The model under review builds one solid part; all positions refer to its coordinate system, in mm. A direction names the side the tool comes from. Round coordinates to 2 decimals unless told otherwise and drop trailing zeros. Use one line per item in the form item = value.
from build123d import *

# Parameters (mm, degrees)
SKETCH1_R            = 180
SKETCH1_R_2          = 110
BOTTOM_ANNULUS_DEPTH = 10
SKETCH3_R            = 180
SKETCH3_R_2          = 110
ANNULUS_PLENUM_DEPTH = 12
SKETCH4_R            = 180
SKETCH4_R_2          = 110
TOP_ANNULUS_DEPTH    = 10
SKETCH8_R            = 6.6
CUT_EXTRUDE1_DEPTH   = 75
SKETCH6_R            = 18
SKETCH6_R_2          = 10
BOSS_EXTRUDE6_DEPTH  = 6.871206759
SKETCH10_R           = 10
SKETCH10_R_2         = 7
BOSS_EXTRUDE7_DEPTH  = 33.989306272


with BuildPart() as part:
    # Sketch1 → Bottom Annulus (new body)
    with BuildSketch(Plane.XY):
        Circle(SKETCH1_R)
        Circle(SKETCH1_R_2, mode=Mode.SUBTRACT)
    extrude(amount=BOTTOM_ANNULUS_DEPTH)

    # Sketch3 → Annulus Plenum (add)
    with BuildSketch(Plane.XY.offset(10)):
        Circle(SKETCH3_R)
        Circle(SKETCH3_R_2, mode=Mode.SUBTRACT)
    extrude(amount=ANNULUS_PLENUM_DEPTH)

    # Sketch4 → Top annulus (add)
    with BuildSketch(Plane.XY.offset(22)):
        Circle(SKETCH4_R)
        Circle(SKETCH4_R_2, mode=Mode.SUBTRACT)
    extrude(amount=TOP_ANNULUS_DEPTH)

    # Sketch8 → Cut-Extrude1 (cut)
    with BuildSketch(Plane.XY.offset(32)):
        with Locations((-37.181108248, 140.450646422)):
            Circle(SKETCH8_R)
        with Locations((38.025538928, 140.224381904)):
            Circle(SKETCH8_R)
        with Locations((103.043273656, 102.425107495)):
            Circle(SKETCH8_R)
        with Locations((140.450646422, 37.181108248)):
            Circle(SKETCH8_R)
        with Locations((140.224381904, -38.025538928)):
            Circle(SKETCH8_R)
        with Locations((102.425107495, -103.043273656)):
            Circle(SKETCH8_R)
        with Locations((37.181108248, -140.450646422)):
            Circle(SKETCH8_R)
        with Locations((-38.025538928, -140.224381904)):
            Circle(SKETCH8_R)
        with Locations((-103.043273656, -102.425107495)):
            Circle(SKETCH8_R)
        with Locations((-140.450646422, -37.181108248)):
            Circle(SKETCH8_R)
        with Locations((-140.224381904, 38.025538928)):
            Circle(SKETCH8_R)
        with Locations((-102.425107495, 103.043273656)):
            Circle(SKETCH8_R)
    extrude(amount=-CUT_EXTRUDE1_DEPTH, mode=Mode.SUBTRACT)

    # Sketch6 → Boss-Extrude6 (add)
    # profile 1 of 12: a face of its own
    with BuildSketch(Plane.XY.offset(32)):
        with Locations((0, 145)):
            Circle(SKETCH6_R)
        with Locations((0, 145)):
            Circle(SKETCH6_R_2, mode=Mode.SUBTRACT)
    # profile 2 of 12: a face of its own
    with BuildSketch(Plane.XY.offset(32)):
        with Locations((72.5, 125.573683549)):
            Circle(SKETCH6_R)
        with Locations((72.5, 125.573683549)):
            Circle(SKETCH6_R_2, mode=Mode.SUBTRACT)
    # profile 3 of 12: a face of its own
    with BuildSketch(Plane.XY.offset(32)):
        with Locations((125.573683549, 72.5)):
            Circle(SKETCH6_R)
        with Locations((125.573683549, 72.5)):
            Circle(SKETCH6_R_2, mode=Mode.SUBTRACT)
    # profile 4 of 12: a face of its own
    with BuildSketch(Plane.XY.offset(32)):
        with Locations((145, 0)):
            Circle(SKETCH6_R)
        with Locations((145, 0)):
            Circle(SKETCH6_R_2, mode=Mode.SUBTRACT)
    # profile 5 of 12: a face of its own
    with BuildSketch(Plane.XY.offset(32)):
        with Locations((125.573683549, -72.5)):
            Circle(SKETCH6_R)
        with Locations((125.573683549, -72.5)):
            Circle(SKETCH6_R_2, mode=Mode.SUBTRACT)
    # profile 6 of 12: a face of its own
    with BuildSketch(Plane.XY.offset(32)):
        with Locations((72.5, -125.573683549)):
            Circle(SKETCH6_R)
        with Locations((72.5, -125.573683549)):
            Circle(SKETCH6_R_2, mode=Mode.SUBTRACT)
    # profile 7 of 12: a face of its own
    with BuildSketch(Plane.XY.offset(32)):
        with Locations((0, -145)):
            Circle(SKETCH6_R)
        with Locations((0, -145)):
            Circle(SKETCH6_R_2, mode=Mode.SUBTRACT)
    # profile 8 of 12: a face of its own
    with BuildSketch(Plane.XY.offset(32)):
        with Locations((-72.5, -125.573683549)):
            Circle(SKETCH6_R)
        with Locations((-72.5, -125.573683549)):
            Circle(SKETCH6_R_2, mode=Mode.SUBTRACT)
    # profile 9 of 12: a face of its own
    with BuildSketch(Plane.XY.offset(32)):
        with Locations((-125.573683549, -72.5)):
            Circle(SKETCH6_R)
        with Locations((-125.573683549, -72.5)):
            Circle(SKETCH6_R_2, mode=Mode.SUBTRACT)
    # profile 10 of 12: a face of its own
    with BuildSketch(Plane.XY.offset(32)):
        with Locations((-145, 0)):
            Circle(SKETCH6_R)
        with Locations((-145, 0)):
            Circle(SKETCH6_R_2, mode=Mode.SUBTRACT)
    # profile 11 of 12: a face of its own
    with BuildSketch(Plane.XY.offset(32)):
        with Locations((-125.573683549, 72.5)):
            Circle(SKETCH6_R)
        with Locations((-125.573683549, 72.5)):
            Circle(SKETCH6_R_2, mode=Mode.SUBTRACT)
    # profile 12 of 12: a face of its own
    with BuildSketch(Plane.XY.offset(32)):
        with Locations((-72.5, 125.573683549)):
            Circle(SKETCH6_R)
        with Locations((-72.5, 125.573683549)):
            Circle(SKETCH6_R_2, mode=Mode.SUBTRACT)
    extrude(amount=BOSS_EXTRUDE6_DEPTH)

    # Sketch10 → Boss-Extrude7 (add)
    # profile 1 of 12: a face of its own
    with BuildSketch(Plane.XY.offset(32)):
        with Locations(Location((0, 145, 0), (0, 0, 180))):
            Circle(SKETCH10_R)
        with Locations(Location((0, 145, 0), (0, 0, 180))):
            Circle(SKETCH10_R_2, mode=Mode.SUBTRACT)
    # profile 2 of 12: a face of its own
    with BuildSketch(Plane.XY.offset(32)):
        with Locations(Location((72.5, 125.573683549, 0), (0, 0, 180))):
            Circle(SKETCH10_R)
        with Locations(Location((72.5, 125.573683549, 0), (0, 0, 180))):
            Circle(SKETCH10_R_2, mode=Mode.SUBTRACT)
    # profile 3 of 12: a face of its own
    with BuildSketch(Plane.XY.offset(32)):
        with Locations(Location((125.573683549, 72.5, 0), (0, 0, 180))):
            Circle(SKETCH10_R)
        with Locations(Location((125.573683549, 72.5, 0), (0, 0, 180))):
            Circle(SKETCH10_R_2, mode=Mode.SUBTRACT)
    # profile 4 of 12: a face of its own
    with BuildSketch(Plane.XY.offset(32)):
        with Locations(Location((145, 0, 0), (0, 0, 180))):
            Circle(SKETCH10_R)
        with Locations(Location((145, 0, 0), (0, 0, 180))):
            Circle(SKETCH10_R_2, mode=Mode.SUBTRACT)
    # profile 5 of 12: a face of its own
    with BuildSketch(Plane.XY.offset(32)):
        with Locations(Location((125.573683549, -72.5, 0), (0, 0, 180))):
            Circle(SKETCH10_R)
        with Locations(Location((125.573683549, -72.5, 0), (0, 0, 180))):
            Circle(SKETCH10_R_2, mode=Mode.SUBTRACT)
    # profile 6 of 12: a face of its own
    with BuildSketch(Plane.XY.offset(32)):
        with Locations(Location((72.5, -125.573683549, 0), (0, 0, 180))):
            Circle(SKETCH10_R)
        with Locations(Location((72.5, -125.573683549, 0), (0, 0, 180))):
            Circle(SKETCH10_R_2, mode=Mode.SUBTRACT)
    # profile 7 of 12: a face of its own
    with BuildSketch(Plane.XY.offset(32)):
        with Locations(Location((0, -145, 0), (0, 0, 180))):
            Circle(SKETCH10_R)
        with Locations(Location((0, -145, 0), (0, 0, 180))):
            Circle(SKETCH10_R_2, mode=Mode.SUBTRACT)
    # profile 8 of 12: a face of its own
    with BuildSketch(Plane.XY.offset(32)):
        with Locations(Location((-72.5, -125.573683549, 0), (0, 0, 180))):
            Circle(SKETCH10_R)
        with Locations(Location((-72.5, -125.573683549, 0), (0, 0, 180))):
            Circle(SKETCH10_R_2, mode=Mode.SUBTRACT)
    # profile 9 of 12: a face of its own
    with BuildSketch(Plane.XY.offset(32)):
        with Locations(Location((-125.573683549, -72.5, 0), (0, 0, 180))):
            Circle(SKETCH10_R)
        with Locations(Location((-125.573683549, -72.5, 0), (0, 0, 180))):
            Circle(SKETCH10_R_2, mode=Mode.SUBTRACT)
    # profile 10 of 12: a face of its own
    with BuildSketch(Plane.XY.offset(32)):
        with Locations(Location((-145, 0, 0), (0, 0, 180))):
            Circle(SKETCH10_R)
        with Locations(Location((-145, 0, 0), (0, 0, 180))):
            Circle(SKETCH10_R_2, mode=Mode.SUBTRACT)
    # profile 11 of 12: a face of its own
    with BuildSketch(Plane.XY.offset(32)):
        with Locations(Location((-125.573683549, 72.5, 0), (0, 0, 180))):
            Circle(SKETCH10_R)
        with Locations(Location((-125.573683549, 72.5, 0), (0, 0, 180))):
            Circle(SKETCH10_R_2, mode=Mode.SUBTRACT)
    # profile 12 of 12: a face of its own
    with BuildSketch(Plane.XY.offset(32)):
        with Locations(Location((-72.5, 125.573683549, 0), (0, 0, 180))):
            Circle(SKETCH10_R)
        with Locations(Location((-72.5, 125.573683549, 0), (0, 0, 180))):
            Circle(SKETCH10_R_2, mode=Mode.SUBTRACT)
    extrude(amount=BOSS_EXTRUDE7_DEPTH)


solid = part.part
(1) Insertion check: P1, Ø11, axis at x = 69.5, y = 128, coming from the +Z side; P2, Ø11, axis at x = 145, y = 0, coming from the +Z side; P3, Ø2, axis at x = 23.5, z = 22.5, coming from the +Y side; P4, Ø10.5, axis at x = 38.03, y = 140.22, coming from the -Z side. Each pin has a flat end and moves straight along its axis. Give the tip position at first contact, or say it passes through.
Geometry results:
P1 = 65.99
P2 = 32
P3 = 178.59
P4 = through
(2) Machinability: for faces 3 (the cylindrical face through (-127.917, 90.347, 35.388)), 4 (the cylindrical face through (-103.86, 96.6, 16.22)), which of the approach directions +Z, -Z, +X, -X, +Y, -Y give a long, thin tool a straight path to every point of the face, cutting with its end or side? Answer none if there is none.
Geometry results:
face_3 = +Z
face_4 = +Z, -Z
(3) To check wall thickness, follow L1, parallel to X at y = -72.5, z = 40; L2, parallel to Y at x = 37, z = 30. State the ranges of each line that lie inside material, in increasing order.
Geometry results:
L1 = -135.57 to -132.57, -118.57 to -115.57, 115.57 to 118.57, 132.57 to 135.57
L2 = -176.16 to -147.05, -133.85 to -103.59, 103.59 to 133.7, 146.74 to 176.16
(4) The part is to be moulded in two halves that separate along X. For faces 1 (the cylindrical face through (-134.354, -39.709, 16.224)), 2 (the flat face through (-147, -7, 65.989)), say which applies: +X half, -X half, draft (parallel to the pull), parting line (faces both ways), or undercut.
Geometry results:
face_1 = undercut
face_2 = draft
(5) Add section C-C on z = 23. Count the separate pieces of the cut face and the enclosed holes in it, then the cut area to 3 significant figures.
Geometry results:
separate_pieces = 1
enclosed_holes = 13
area = 62,100 mm2
